Geometry check sheet. Reference: the model listing, model coordinates, mm. A direction names the side the tool comes from. Coordinates: 2 decimals unless noted, no trailing zeros. Write each loop counter-clockwise with the first axis right and the second up, starting at its lowest first coordinate (ties: lowest second). Pieces come first, ordered by that corner, then holes. Notation, with made-up numbers: (18, 61) -> (28, 61) arc R23 cw to (28, 83) -> close; hole circle Ø9 at (-18.75, -39.5). An arc over 180 degrees is marked (long way). Put each result on its own line as item: value. Start each with the question number.
from build123d import *

# Parameters (mm, degrees)
SKETCH_1_W               = 50
SKETCH_1_H               = 85
EXTRUDE_1_DEPTH          = 5
SKETCH_2_W               = 5
SKETCH_2_H               = 20
EXTRUDE_2_DEPTH          = 5
PATTERN_LINEAR_1_COUNT   = 2
PATTERN_LINEAR_1_PITCH   = 40
MIRROR_1_COPY_1_SKETCH_W = 5
MIRROR_1_COPY_1_SKETCH_H = 20
MIRROR_1_COPY_1_DEPTH    = 5
SKETCH_4_W               = 20
SKETCH_4_H               = 5
EXTRUDE_3_DEPTH          = 5


with BuildPart() as part:
    # 스케치1 → 보스-돌출1 (new body)
    with BuildSketch(Plane.XY):
        Rectangle(SKETCH_1_W, SKETCH_1_H)
    extrude(amount=EXTRUDE_1_DEPTH)

    # 스케치2 → 보스-돌출2 (add)
    with BuildSketch(Plane.XY.offset(5)):
        with Locations((-27.5, -12.5)):
            Rectangle(SKETCH_2_W, SKETCH_2_H)
    extrude_2 = extrude(amount=-EXTRUDE_2_DEPTH)

    # 선형 패턴1: 보스-돌출2 ×2
    with Locations(*[(0, i * PATTERN_LINEAR_1_PITCH, 0) for i in range(1, PATTERN_LINEAR_1_COUNT)]):
        add(extrude_2)

    # 대칭 복사1: 보스-돌출2 across plane
    add(extrude_2.mirror(Plane(origin=(0, 0, 0), x_dir=(0, 0, 1), z_dir=(1, 0, 0))))

    # 대칭 복사1 copy 1 sketch → 대칭 복사1 copy 1 (add)
    with BuildSketch(Plane(origin=(0, 40, 5), x_dir=(-1, 0, 0), z_dir=(0, 0, 1))):
        with Locations((-27.5, 12.5)):
            Rectangle(MIRROR_1_COPY_1_SKETCH_W, MIRROR_1_COPY_1_SKETCH_H)
    extrude(amount=-MIRROR_1_COPY_1_DEPTH)

    # 스케치4 → 보스-돌출3 (add)
    with BuildSketch(Plane.XY.offset(5)):
        with Locations((0, 45)):
            Rectangle(SKETCH_4_W, SKETCH_4_H)
    extrude(amount=-EXTRUDE_3_DEPTH)


solid = part.part
Item 1: Section check D-D, the plane x = -21. Enter the section's corners in (y, z).
Item 2: Go/stop test with flat-tipped pins: P1, Ø1.5, axis at x = 26.5, z = 2.5, coming from the -Y side; P2, Ø1.5, axis at x = 27, z = 3.5, coming from the +Y side; P3, Ø2, axis at x = 17, z = 0.5, coming from the +Y side. Record where each tip stops, or that it passes through.
Item 3: Section check B-B, the plane z = 3.4. Enter the section's corners in (x, y).
Item 4: Access from +Z, -Z, +X, -X, +Y, -Y to the whole of each face (thin tool, end or side, straight path). Record for faces 1 (the flat face through (28, 17.5, 3)), 2 (the flat face through (25, -33, 2)), 3 (the flat face through (-28, 37.5, 3)), 4 (the flat face through (-28, -2.5, 3)), 5 (the flat face through (17, 42.5, 2)).
Item 5: Mould release check, pull along Y, two halves, no side actions. Record for faces 6 (the flat face through (-28, 17.5, 3)), 7 (the flat face through (0, 47.5, 3)), 8 (the flat face through (0, 3, 0)), 9 (the flat face through (25, 7, 2)): released by +Y, released by -Y, zero draft, split by the parting line, or undercut.
Item 6: Section check A-A, the plane x = 26. Enter the section's corners in (y, z), and give its area (3 significant figures).
Item 7: Scan lines: line 1 along X through (y, z) = (3, 2.1); line 2 along Y through (x, z) = (19, 2.9). Record each from-to range of solid material in increasing order. Write a range as [from, to].
Item 8: Section check C-C, the plane y = 8. Enter the section's corners in (x, z).
From the geometry:
1. outline: (-42.5, 0) -> (42.5, 0) -> (42.5, 5) -> (-42.5, 5) -> close
2. P1: y = -22.5
2. P2: y = 37.5
2. P3: y = 42.5
3. outline: (-30, -22.5) -> (-25, -22.5) -> (-25, -42.5) -> (25, -42.5) -> (25, -22.5) -> (30, -22.5) -> (30, -2.5) -> (25, -2.5) -> (25, 17.5) -> (30, 17.5) -> (30, 37.5) -> (25, 37.5) -> (25, 42.5) -> (10, 42.5) -> (10, 47.5) -> (-10, 47.5) -> (-10, 42.5) -> (-25, 42.5) -> (-25, 37.5) -> (-30, 37.5) -> (-30, 17.5) -> (-25, 17.5) -> (-25, -2.5) -> (-30, -2.5) -> close
4. face 1: +Z, -Z, +X
4. face 2: +Z, -Z, +X, -Y
4. face 3: +Z, -Z, -X, +Y
4. face 4: +Z, -Z, -X
4. face 5: +Z, -Z, +X, +Y
5. face 6: undercut
5. face 7: released by +Y
5. face 8: zero draft
5. face 9: undercut
6. outline: (-22.5, 0) -> (-2.5, 0) -> (-2.5, 5) -> (-22.5, 5) -> close; (17.5, 0) -> (37.5, 0) -> (37.5, 5) -> (17.5, 5) -> close
6. area: 200 mm²
7. line 1: [-25, 25]
7. line 2: [-42.5, 42.5]
8. outline: (-25, 0) -> (25, 0) -> (25, 5) -> (-25, 5) -> close
